from build123d import *

# Parameters (mm, degrees)
PEDAL_COVER_DEPTH       = 2.5
SKETCH2_R               = 1.65
COVER_SCREW_HOLES_DEPTH = 112.685719768


with BuildPart() as part:
    # Sketch1 → Pedal cover (new body)
    with BuildSketch(Plane(origin=(0, 28, 0), x_dir=(1, 0, 0), z_dir=(0, 1, 0))):
        Polygon((86.3, 45.2), (84.9, 45), (83.6, 44.4), (82.1, 42.9), (81.5, 41.6), (81.3, 40.2), (81.5, 38.8), (82.3, 37.3), (82.2, 37.2), (69.7, 37.2), (71.1, 32.3), (72.4, 25.5), (73, 20.7), (73.6, 12.1), (73.7, 1.7), (73.4, -5.3), (72.5, -13.4), (71.3, -19.5), (70.2, -23.8), (69.1, -27.1), (82.2, -27.1), (82.3, -27.2), (81.5, -28.7), (81.3, -30.1), (81.5, -31.5), (82.1, -32.8), (83.6, -34.3), (84.9, -34.9), (86.3, -35.1), (87.7, -34.9), (89, -34.3), (90.5, -32.8), (91.1, -31.5), (91.3, -30.1), (91.1, -28.7), (90.3, -27.2), (90.4, -27.1), (92.2, -27.1), (96.8, -26.1), (98.7, -24.7), (99.7, -23.7), (101.1, -21.8), (102.1, -17.2), (102.1, 27.3), (101.1, 31.9), (99.7, 33.8), (98.7, 34.8), (96.8, 36.2), (92.2, 37.2), (90.4, 37.2), (90.3, 37.3), (91.1, 38.8), (91.3, 40.2), (91.1, 41.6), (90.5, 42.9), (89, 44.4), (87.7, 45), align=None)
    extrude(amount=PEDAL_COVER_DEPTH)

    # Sketch2 → Cover screw holes (cut, through all)
    with BuildSketch(Plane(origin=(0, 28, 0), x_dir=(1, 0, 0), z_dir=(0, 1, 0))):
        with Locations(Location((86.28, 40.2, 0), (0, 0, 270))):
            Circle(SKETCH2_R)
        with Locations(Location((86.28, -30.1, 0), (0, 0, 270))):
            Circle(SKETCH2_R)
    extrude(amount=COVER_SCREW_HOLES_DEPTH, mode=Mode.SUBTRACT)


solid = part.part
Here's how the part is built. I have some questions about the finished solid (model axes, mm). A direction names the side the tool comes from. Round coordinates to 2 decimals unless told otherwise and drop trailing zeros. Loops run counter-clockwise (first coordinate to the right, second up) from the corner with the lowest first, then second, coordinate; pieces in that order, holes last. Notation, with made-up numbers: (12.25, 48) -> (43.25, 48) arc R20 ccw to (43.25, 63) -> close; hole circle Ø3 at (23, -23.5). An arc over 180 degrees is marked (long way). Write each question's results on one line, items separated by ' | '.
(1) If I drill on L1, parallel to Z at x = 86.28, y = 29.4; L2, parallel to X at y = 28.9, z = -40.2; L3, parallel to Z at x = 82, y = 30.2, over which ranges is the centre line in solid material (lowest first)?
Worked answers:
L1: -45.2 to -41.85, -38.55 to 28.45, 31.75 to 35.1 | L2: 81.3 to 84.63, 87.93 to 91.3 | L3: -42.68 to -37.86, -37.2 to 27.1, 27.76 to 32.58
(2) For P1, Ø0.8, axis at x = 74.5, y = 28.5, coming from the +Z side, with a flat end and sliding along its axis, tell me the tip position at first contact or that it passes through.
Worked answers:
P1: z = 27.1
(3) If we section it at B-B, the plane y = 28.5: Give the number of separate pieces and of enclosed holes in the cut face, then the cut area to 3 significant figures.
Worked answers:
separate pieces: 1 | enclosed holes: 2 | area: 1,980 mm2
(4) For faces 1 (the face through (94.5, 29.2, -36.7)), 2 (the face through (72.7, 29.2, -23.1)), 3 (the face through (91, 29, -37.2)), which set-ups out of +Z, -Z, +X, -X, +Y, -Y let a thin tool reach every point of the face, with its end or its side?
Worked answers:
face 1: -Z, +X, +Y, -Y | face 2: -X, +Y, -Y | face 3: +X, +Y, -Y
(5) If we section it at A-A, the plane x = 76: List the corners of the cut face in (y, z) for me.
Worked answers:
outline: (28, -37.2) -> (30.5, -37.2) -> (30.5, 27.1) -> (28, 27.1) -> close
(6) If we section it at C-C, the plane z = -33: List the corners of the cut face in (x, y) for me.
Worked answers:
outline: (70.9, 28) -> (100.29, 28) -> (100.29, 30.5) -> (70.9, 30.5) -> close
